Work out the finished part from the listing and answer in its coordinate system (mm). A direction names the side the tool comes from. Round coordinates to 2 decimals unless told otherwise and drop trailing zeros. Loops run counter-clockwise (first coordinate to the right, second up) from the corner with the lowest first, then second, coordinate; pieces in that order, holes last. Notation, with made-up numbers: (65.25, 79.5) -> (80.25, 79.5) arc R18 ccw to (80.25, 109.5) -> close; hole circle Ø11 at (58.5, -4.75). An arc over 180 degrees is marked (long way). Use one line per item in the form item = value.
Autodesk Inventor part; units mm, degrees
ref_plane "YZ Plane" through (0, 0, 0) normal (1, 0, 0) x (0, 1, 0)
ref_plane "XZ Plane" through (0, 0, 0) normal (0, 1, 0) x (-1, 0, 0)
ref_plane "XY Plane" through (0, 0, 0) normal (0, 0, 1) x (1, 0, 0)
sketch "Skizze1" plane through (0, 0, 0) normal (0, 0, 1) x (1, 0, 0)
  line L0 (-80, 25) -> (80, 25)
  line L1 (80, 25) -> (80, -65)
  line L2 (80, -65) -> (-80, -65)
  line L3 (-80, -65) -> (-80, 25)
  line L4 (-112, 0) -> (112, 0)
  line L5 (0, -83) -> (0, 43)
  circle A0 centre (-30, 0) radius 2.7
  circle A1 centre (30, 0) radius 2.7
  point P0 (0, 0)
  dimension "d0" = 25
  dimension "d1" = 160
  dimension "d2" = 60
  dimension "d3" = 5.4
  dimension "d4" = 90
extrude "Extrusion1" add sketch "Skizze1" along normal blind 10 contours L0 L5 L4 A0 L3 | L0 L1 L4 A1 L5 | L4 A0 L5 L2 L3 | L4 A1 L1 L2 L5
sketch "Skizze2" plane through (0, 0, 0) normal (0, 0, -1) x (-1, 0, 0)
  circle A0 centre (-30, 0) radius 2.7
  circle A1 centre (30, 0) radius 2.7
  circle A2 centre (-30, 0) radius 7
  circle A3 centre (30, 0) radius 7
  point P0 (0, 0)
  dimension "d7" = 14
extrude "Extrusion2" cut sketch "Skizze2" against normal blind 6
sketch "Skizze3" plane through (0, 0, 0) normal (0, 0, -1) x (-1, 0, 0)
  circle A0 centre (12.5, -59) radius 2.067
  circle A1 centre (-12.5, -59) radius 2.067
  circle A2 centre (-12.5, -37) radius 2.067
  circle A3 centre (12.5, -37) radius 2.067
  line L0 (30, -31) -> (30, -65)
  line L1 (30, -65) -> (-30, -65)
  line L2 (-30, -65) -> (-30, -31)
  line L3 (-30, -31) -> (30, -31)
  line L4 (-30, -48) -> (30, -48)
  line L5 (0, -31) -> (0, -65)
  circle A4 centre (-20, -48) radius 2.067
  circle A5 centre (20, -48) radius 2.067
  point P0 (0, 0)
  point P1 (-20, -48)
  point P2 (20, -48)
  dimension "d10" = 40
hole "Bohrung1" at (20, -48, 0) at (-20, -48, 0) direction (0, 0, 1) diameter 5.5 end through all counterbore diameter 10 counterbore depth 5.4
sketch "Skizze4" plane through (-80, 25, 0) normal (0, 1, 0) x (1, 0, 0)
  line L0 (0, -10) -> (160, -10)
  line L1 (160, 0) -> (160, -10)
  line L2 (0, 0) -> (0, -10)
  line L3 (160, -5) -> (0, -5)
  line L4 (80, 0) -> (80, -10)
  point P0 (155, -5)
  point P1 (145, -5)
  point P2 (5, -5)
  point P3 (15, -5)
  dimension "d18" = 5
  dimension "d19" = 10
hole "Bohrung2" at (75, 25, 5) at (65, 25, 5) at (-75, 25, 5) at (-65, 25, 5) direction (0, -1, 0) diameter 2.459 depth 10 tip angle 118
sketch "Skizze5" plane through (0, 0, 10) normal (0, 0, 1) x (1, 0, 0)
  line L0 (80, 25) -> (80, -65)
  line L1 (-80, 25) -> (80, 25)
  line L2 (-80, -65) -> (-80, 25)
  line L3 (80, -65) -> (-80, -65)
  line L4 (0, -65) -> (0, 25)
  line L5 (-80, -20) -> (80, -20)
  line L6 (-65, 5) -> (65, 5)
  line L7 (65, 5) -> (65, -45)
  line L8 (65, -45) -> (-65, -45)
  line L9 (-65, -45) -> (-65, 5)
  point P0 (0, 0)
  dimension "d27" = 130
  dimension "d28" = 50
hole "Bohrung3" at (-65, 5, 10) at (65, 5, 10) at (65, -45, 10) at (-65, -45, 10) direction (0, 0, -1) diameter 4.5 end through all counterbore diameter 8 counterbore depth 6
properties part number "1_0204_010"
(1) For a pull along Y with two mould halves and no side action, classify faces 1 (the flat face through (-63, 3, 4)), 2 (the flat face through (80, -19, 5)), 3 (the flat face through (1, -65, 5)) as +Y half, -Y half, draft (parallel to the pull), parting line (faces both ways), or undercut.
Completed:
face_1 = undercut
face_2 = draft
face_3 = -Y half
(2) Consider L1, parallel to Y at x = -65, z = 2.55; L2, parallel to X at y = -48, z = 3.05; L3, parallel to X at y = 5, z = 6.05. Determine where each line is inside the solid, lowest interval first.
Completed:
L1 = -65 to -47.25, -42.75 to 2.75, 7.25 to 25
L2 = -80 to -25, -15 to 15, 25 to 80
L3 = -80 to -69, -61 to 61, 69 to 80
(3) Given P1, Ø18, axis at x = -30, y = 0, coming from the +Z side; P2, Ø8.5, axis at x = 30, y = 0, coming from the -Z side, each flat-ended and moving along its own axis, determine where each tip first touches the part or whether it passes through.
Completed:
P1 = 10
P2 = 6
(4) Find section B-B, the plane y = 5. Write down the section's boundary in (x, z), then the cut area to 3 significant figures.
Completed:
outline = (-80, 0) -> (-67.25, 0) -> (-67.25, 4) -> (-69, 4) -> (-69, 10) -> (-80, 10) -> close; (-62.75, 0) -> (-34.9, 0) -> (-34.9, 6) -> (-25.1, 6) -> (-25.1, 0) -> (25.1, 0) -> (25.1, 6) -> (34.9, 6) -> (34.9, 0) -> (62.75, 0) -> (62.75, 4) -> (61, 4) -> (61, 10) -> (-61, 10) -> (-61, 4) -> (-62.75, 4) -> close; (67.25, 0) -> (80, 0) -> (80, 10) -> (69, 10) -> (69, 4) -> (67.25, 4) -> close
area = 1,350 mm2
(5) For faces 4 (the flat face through (-17.8, -45.8, 5.4)), 5 (the flat face through (67, -47, 4)), 6 (the cylindrical face through (67.196, -44.512, 1.972)), determine the directions among +Z, -Z, +X, -X, +Y, -Y from which every point of the face is accessible in a straight line to the end or side of a thin tool.
Completed:
face_4 = -Z
face_5 = +Z
face_6 = +Z, -Z
(6) Find section A-A, the plane x = 20. Write down the section's boundary in (y, z).
Completed:
outline = (-65, 0) -> (-53, 0) -> (-53, 5.4) -> (-50.75, 5.4) -> (-50.75, 10) -> (-65, 10) -> close; (-45.25, 5.4) -> (-43, 5.4) -> (-43, 0) -> (25, 0) -> (25, 10) -> (-45.25, 10) -> close
